from build123d import *

# Parameters (mm, degrees)
F_3_8_16_TAPPED_HOLE1_D     = 7.9375
F_3_8_16_TAPPED_HOLE1_DEPTH = 29.5402
F_3_8_16_TAPPED_HOLE1_TIP   = 2.384665582
CHAMFER1_SIZE               = 0.762
FILLET1_R                   = 0.381
SKETCH4_R                   = 1.5875
CUT_EXTRUDE1_DEPTH          = 27.94


with BuildPart() as part:
    # Sketch1 → Revolve1 (revolve)
    with BuildSketch(Plane.XY, mode=Mode.PRIVATE) as revolve1_sk:
        Polygon((0, 0), (28.575, 0), (28.575, 6.35), (25.4, 6.35), (25.4, 124.46), (0, 124.46), align=None)
    revolve(revolve1_sk.sketch.rotate(Axis((0, 0, 0), (0, 1, 0)), 90), axis=Axis((0, 0, 0), (0, 1, 0)))  # turned: the seam where the file's is

    # 3/8-16 Tapped Hole1
    with Locations(Plane.ZX.offset(124.46)):
        with Locations((0, 0)):
            Hole(F_3_8_16_TAPPED_HOLE1_D / 2, depth=F_3_8_16_TAPPED_HOLE1_DEPTH)
            with Locations((0, 0, -(F_3_8_16_TAPPED_HOLE1_DEPTH + F_3_8_16_TAPPED_HOLE1_TIP / 2))):  # 118° drill point
                Cone(0, F_3_8_16_TAPPED_HOLE1_D / 2, F_3_8_16_TAPPED_HOLE1_TIP, mode=Mode.SUBTRACT)

    # Chamfer1
    chamfer1_edges = [part.edges().sort_by_distance(p)[0] for p in [
        (0, 124.46, 25.4),
    ]]
    chamfer(chamfer1_edges, length=CHAMFER1_SIZE)

    # Fillet1
    fillet1_edges = [part.edges().sort_by_distance(p)[0] for p in [
        (0, 6.35, 25.4),
    ]]
    fillet(fillet1_edges, radius=FILLET1_R)

    # Sketch4 → Cut-Extrude1 (cut)
    with BuildSketch(Plane.XY):
        with Locations((0, 94.9198)):
            Circle(SKETCH4_R)
    extrude(amount=-CUT_EXTRUDE1_DEPTH, mode=Mode.SUBTRACT)


solid = part.part
Source: CAD feature listing. Evaluate the final solid. Frame: model axes, mm. A direction names the side the tool comes from. Round coordinates to 2 decimals unless told otherwise and drop trailing zeros. Loops run counter-clockwise (first coordinate to the right, second up) from the corner with the lowest first, then second, coordinate; pieces in that order, holes last.
Q1. Section A-A, the plane y = 104.5. Return loops of the section in (x, z), plus the area to 3 significant figures.
Q2. Mould query, pull axis Z, two halves, no side actions, for faces 3 (the face through (-0.34, 93.37, -13.19)), 4 (the face through (15.456, 66.033, 20.157)), 5 (the face through (-3.874, 109.483, 0.86)). Classes: pulls with the +Z half, pulls with the -Z half, needs draft (parallel to the pull), parting line crosses it, or undercut.
Q3. Access query for faces 1 (the face through (-1.256, 3.219, 28.547)), 2 (the face through (-26, 6.35, 4)). Directions: +Z, -Z, +X, -X, +Y, -Y. A direction counts if a zero-diameter tool reaches every point of the face in a straight line with its end or side. Return the directions, or none.
Q4. Section B-B, the plane y = 58. Return loops of the section in (x, z).
Q5. Ray query, line 1 (Y direction, x = 0, z = -6); line 2 (X direction, y = 115.5, z = 0); line 3 (Y direction, x = -22, z = -16). Return the intervals inside material, ascending.
Q6. First-contact query: P1, Ø6, axis at y = 88, z = 21.5, coming from the -X side; P2, Ø10.5, axis at x = 0, z = 0, coming from the +Y side; P3, Ø6, axis at y = 83.5, z = 16, coming from the -X side; P4, Ø3.5, axis at x = 0, y = 94.92, coming from the -Z side. Flat tips, straight axial feed; report the tip coordinate or a pass-through.
Solutions:
1. outline: circle Ø50.8 at (0, 0); hole circle Ø7.94 at (0, 0)
1. area: 1,980 mm2
2. face 3: needs draft
2. face 4: parting line crosses it
2. face 5: undercut
3. face 1: +Y, -Y
3. face 2: +Y
4. outline: circle Ø50.8 at (0, 0)
5. line 1: y = 0 to 93.33, 96.51 to 124.46
5. line 2: x = -25.4 to -3.97, 3.97 to 25.4
5. line 3: y = 0 to 6.35
6. P1: stops at x = -17.4
6. P2: stops at y = 124.46
6. P3: stops at x = -21.82
6. P4: stops at z = -25.4
